Design review of the part shown in the three views and the two pictorial views. Dimensions are in mm from the part's minimum x, y and z. A direction names the side the tool comes from. Round coordinates to 2 decimals unless told otherwise and drop trailing zeros. Loops run counter-clockwise (first coordinate to the right, second up) from the corner with the lowest first, then second, coordinate; pieces in that order, holes last. Notation, with made-up numbers: M 24,-21.75 L 35,-21.75 A34 cw 35,15.25 Z; hole C 7,-7.5 d4. An arc over 180 degrees is marked long. Return JSON: item names as keys, results as strings. Group by question number.
Q1. To check wall thickness, follow line 1 along Y through (x, z) = (107, 33.5); line 2 along X through (y, z) = (39, 62.5) (1 decimal); line 3 along X through (y, z) = (39.5, 121) (1 decimal). State the ranges of each line that lie inside material, in increasing order.
Q2. Consider section D-D (y = 15). State the section outline as (x, z) points.
Q3. Consider section B-B (x = 85.5). State the section outline as (y, z) points.
Q4. Consider section C-C (y = 45). State the section outline as (x, z) points (1 decimal), and give its area (3 significant figures).
Q5. Clearance check with flat-ended pins moving along their axes: pin 1 Ø12 at (x, z) = (85.5, 31) entering from -Y; pin 2 Ø8 at (y, z) = (30, 45) entering from +X; pin 3 Ø10 at (y, z) = (41.5, 86.5) entering from -X; pin 4 Ø3 at (x, y) = (93.5, 29) entering from -Z (1 decimal). State where each tip first meets the part, or that it passes through.
Q6. Consider section A-A (z = 39). State the section outline as (x, y) points (1 decimal), and give its area (3 significant figures).
Q7. For the marked faces 1 and 2, list the 3-axis set-ups (+Z, -Z, +X, -X, +Y, -Y) from which the entire face can be reached by the end or side of a thin tool; tool diameter is ignored.
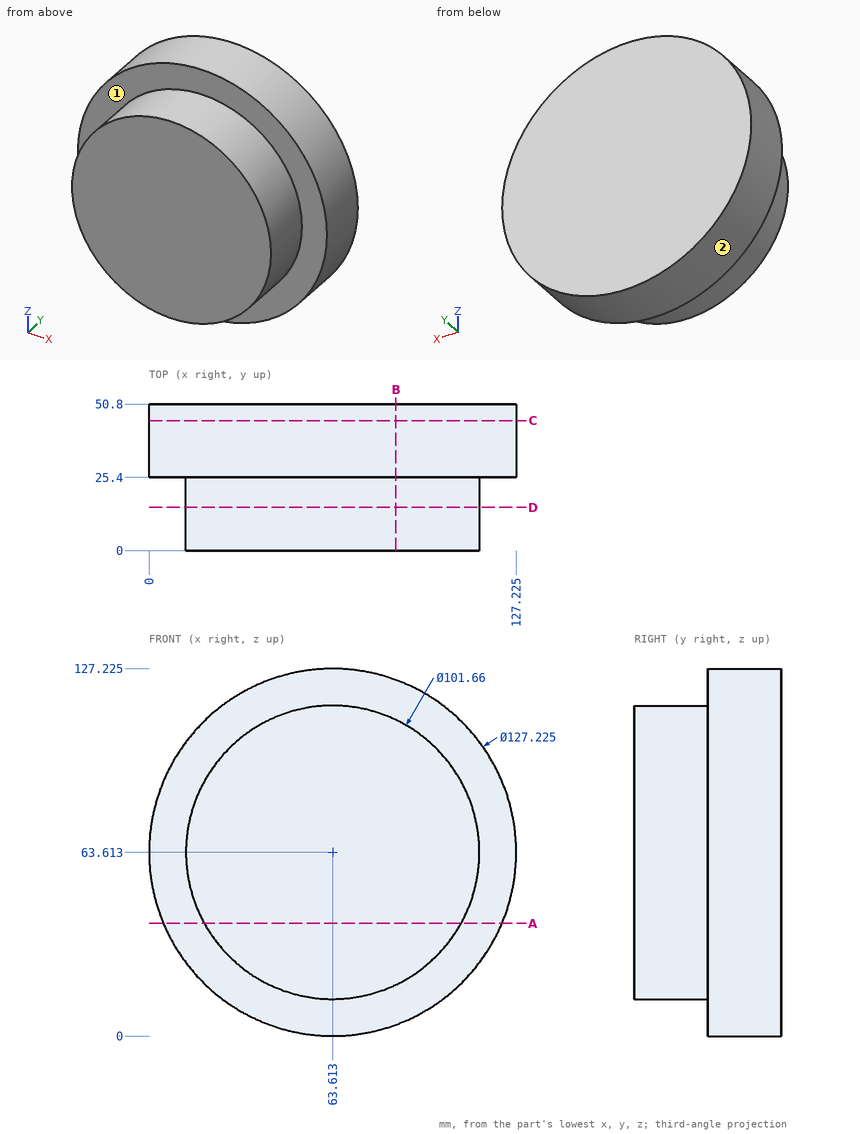
Values:
{
 "1": {"line 1": "y = 25.4 to 50.8", "line 2": "x = 0 to 127.2", "line 3": "x = 36.2 to 91.1"},
 "2": {"outline": "C 63.61,63.61 d101.66"},
 "3": {"outline": "M 0,17.74 L 25.4,17.74 L 25.4,3.88 L 50.8,3.88 L 50.8,123.34 L 25.4,123.34 L 25.4,109.49 L 0,109.49 Z"},
 "4": {"outline": "C 63.6,63.6 d127.2", "area": "12,700 mm2"},
 "5": {"pin 1": "stops at y = 0", "pin 2": "stops at x = 125.52", "pin 3": "stops at x = 2.57", "pin 4": "stops at z = 6.7"},
 "6": {"outline": "M 5,25.4 L 19.1,25.4 L 19.1,0 L 108.1,0 L 108.1,25.4 L 122.3,25.4 L 122.3,50.8 L 5,50.8 Z", "area": "5,240 mm2"},
 "7": {"face 1": "-Y", "face 2": "+Y, -Y"}
}
